Build history of the part. All positions in model axes, mm. A direction names the side the tool comes from. Round coordinates to 2 decimals unless told otherwise and drop trailing zeros. Write each loop counter-clockwise with the first axis right and the second up, starting at its lowest first coordinate (ties: lowest second). Pieces come first, ordered by that corner, then holes. Notation, with made-up numbers: M 55.5,-39 L 79.5,-39 A25 ccw 79.5,-1 Z; hole C 65,56.5 d2. An arc over 180 degrees is marked long. Write item = value, one per line. Start each with the question number.
Q1. Band-saw the part on D-D on z = 70. Write the cut outline in (x, y), plus the area to 3 significant figures.
Q2. Pull direction Y, two halves, no side cores. Call faces 4 (the flat face through (1, 20.32, 51)), 5 (the flat face through (-62.988, -11, 63)), 6 (the flat face through (-56, -32, 48.899)): released by +Y, released by -Y, zero draft, split by the parting line, or undercut.
Q3. Band-saw the part on A-A on z = 64.5. Write the cut outline in (x, y).
Q4. Drop flat-ended pins along their axis: P1, Ø4, axis at y = 0, z = 55, coming from the +X side; P2, Ø3, axis at x = -16.5, y = -22, coming from the +Z side; P3, Ø2.5, axis at x = 33.86, y = 12.7, coming from the -Z side; P4, Ø10, axis at x = 46.5, y = 7.5, coming from the -Z side. Give the stop position or say it passes through.
Q5. Band-saw the part on B-B on y = -33.02. State how many separate pieces and enclosed holes the cut face has, plus the area to 3 significant figures.
Q6. Band-saw the part on C-C on y = -18. Write the cut outline in (x, z), plus the area to 3 significant figures.
Q7. Tool access for faces 1 (the cylindrical face through (36.965, -31.405, 47.695)), 2 (the cylindrical face through (32.71, -34.27, 62.74)), 3 (the flat face through (-52.828, -11, 65)): list every direction of +Z, -Z, +X, -X, +Y, -Y with a clear straight run to the whole face (end or side of a thin tool).
Q8. Probe L1, parallel to X at y = 12.7, z = 48.1; L2, parallel to Z at x = -2.5, y = -18; L3, parallel to X at y = -33, z = 70. List the from-to ranges inside material, lowest first.
```python
from build123d import *

# Parameters (mm, degrees)
BOSS_EXTRUDE1_DEPTH                           = 20.32
BOSS_EXTRUDE1_DEPTH_BACK                      = 40.64
CBORE_FOR_M3_PAN_HEAD_MACHINE_SCREW1_AT_COUNT = 2
CBORE_FOR_M3_PAN_HEAD_MACHINE_SCREW1_AT_PITCH = 91.768246806
CBORE_FOR_M3_PAN_HEAD_MACHINE_SCREW1_2_COUNT  = 2
CBORE_FOR_M3_PAN_HEAD_MACHINE_SCREW1_2_PITCH  = 102.526725891
CBORE_FOR_M3_PAN_HEAD_MACHINE_SCREW1_3_COUNT  = 2
CBORE_FOR_M3_PAN_HEAD_MACHINE_SCREW1_3_PITCH  = 45.72
FILLET1_R                                     = 1.27


with BuildPart() as part:
    # Sketch1 → Boss-Extrude1 (new, two sides: drawn at the far end of the back side and taken through both)
    with BuildSketch(Plane(origin=(0, 0, 0), x_dir=(1, 0, 0), z_dir=(0, 1, 0)).offset(-BOSS_EXTRUDE1_DEPTH_BACK)):
        Polygon((-52.827899024, -76.979185495), (-62.987899024, -76.979185495), (-62.987899024, -46.499185495), (38.940347782, -46.499185495), (64.012100976, -76.979185495), (29.722100976, -76.979185495), (29.722100976, -51.579185495), (-52.827899024, -51.579185495), align=None)
    extrude(amount=BOSS_EXTRUDE1_DEPTH + BOSS_EXTRUDE1_DEPTH_BACK)

    # Sketch4 → CBORE for M3 Pan Head Machine Screw1 (revolve, cut)
    with BuildSketch(Plane(origin=(33.860347782, -33.02, 46.499185495), x_dir=(0, 1, 0), z_dir=(1, 0, 0))):
        Polygon((0, 0), (0, 30.48), (1.7, 30.48), (1.7, 2.4), (3.5, 2.4), (3.5, 0.025), (3.525, 0), align=None)
    cbore_for_m3_pan_head_machine_screw1 = revolve(axis=Axis((33.860347782, -33.02, 40.149185495), (0, 0, 1)), mode=Mode.SUBTRACT)

    # CBORE for M3 Pan Head Machine Screw1 at: CBORE for M3 Pan Head Machine Screw1 ×2
    with Locations(*[(-i * CBORE_FOR_M3_PAN_HEAD_MACHINE_SCREW1_AT_PITCH, 0, 0) for i in range(1, CBORE_FOR_M3_PAN_HEAD_MACHINE_SCREW1_AT_COUNT)]):
        add(cbore_for_m3_pan_head_machine_screw1, mode=Mode.SUBTRACT)

    # CBORE for M3 Pan Head Machine Screw1 2: CBORE for M3 Pan Head Machine Screw1 ×2
    with Locations(*[Vector(-0.8950665888221234, 0.4459325078689913, 0) * (i * CBORE_FOR_M3_PAN_HEAD_MACHINE_SCREW1_2_PITCH) for i in range(1, CBORE_FOR_M3_PAN_HEAD_MACHINE_SCREW1_2_COUNT)]):
        add(cbore_for_m3_pan_head_machine_screw1, mode=Mode.SUBTRACT)

    # CBORE for M3 Pan Head Machine Screw1 3: CBORE for M3 Pan Head Machine Screw1 ×2
    with Locations(*[(0, i * CBORE_FOR_M3_PAN_HEAD_MACHINE_SCREW1_3_PITCH, 0) for i in range(1, CBORE_FOR_M3_PAN_HEAD_MACHINE_SCREW1_3_COUNT)]):
        add(cbore_for_m3_pan_head_machine_screw1, mode=Mode.SUBTRACT)

    # Fillet1
    fillet1_edges = [part.edges().sort_by_distance(p)[0] for p in [
        (-62.987899024, -10.16, 46.499185495),
        (38.940347782, -10.16, 46.499185495),
        (29.722100976, -10.16, 51.579185495),
        (-52.827899024, -10.16, 51.579185495),
    ]]
    fillet(fillet1_edges, radius=FILLET1_R)


solid = part.part
```
Conclusion:
q1.outline = M -62.99,-40.64 L -52.83,-40.64 L -52.83,20.32 L -62.99,20.32 Z; M 29.72,-40.64 L 58.27,-40.64 L 58.27,20.32 L 29.72,20.32 Z; hole C -57.91,-33.02 d3.4; hole C -57.91,12.7 d3.4; hole C 33.86,-33.02 d3.4; hole C 33.86,12.7 d3.4
q1.area = 2,320 mm^2
q2.face_4 = released by +Y
q2.face_5 = zero draft
q2.face_6 = undercut
q3.outline = M -62.99,-40.64 L -52.83,-40.64 L -52.83,20.32 L -62.99,20.32 Z; M 29.72,-40.64 L 53.75,-40.64 L 53.75,20.32 L 29.72,20.32 Z; hole C -57.91,-33.02 d3.4; hole C -57.91,12.7 d3.4; hole C 33.86,-33.02 d3.4; hole C 33.86,12.7 d3.4
q4.P1 = 47.58
q4.P2 = 51.58
q4.P3 = through
q4.P4 = 49.61
q5.separate_pieces = 3
q5.enclosed_holes = 0
q5.area = 1,170 mm^2
q6.outline = M -62.99,47.77 A1.27 ccw -61.72,46.5 L 38.34,46.5 A1.27 ccw 39.32,46.96 L 64.01,76.98 L 29.72,76.98 L 29.72,52.85 A1.27 cw 28.45,51.58 L -51.56,51.58 A1.27 cw -52.83,52.85 L -52.83,76.98 L -62.99,76.98 Z
q6.area = 1,390 mm^2
q7.face_1 = -Z
q7.face_2 = +Z, -Z
q7.face_3 = +Z, +Y, -Y
q8.L1 = -62.99 to -61.41, -54.41 to 30.36, 37.36 to 40.26
q8.L2 = 46.5 to 51.58
q8.L3 = -62.99 to -59.61, -56.21 to -52.83, 29.72 to 32.16, 35.56 to 58.27
